from build123d import *

# Parameters (mm, degrees)
SKETCH1_W           = 66
SKETCH1_H           = 58.3
SKETCH1_R           = 2.05
BOSS_EXTRUDE1_DEPTH = 29
CUT_EXTRUDE1_START  = -29
CUT_EXTRUDE1_DEPTH  = 20
SKETCH6_W           = 10
SKETCH6_H           = 7.9
SKETCH6_R           = 2.05
BOSS_EXTRUDE2_DEPTH = 3
BOSS_EXTRUDE4_DEPTH = 7.9
BOSS_EXTRUDE5_START = -50.4
BOSS_EXTRUDE5_DEPTH = 7.9
CUT_EXTRUDE4_START  = -58.3
SKETCH8_R           = 4.05
CUT_EXTRUDE4_DEPTH  = 58.3
CUT_EXTRUDE5_REACH  = 80.031
SKETCH10_W          = 3
SKETCH10_H          = 6
SKETCH10_W_2        = 4.2
SKETCH10_W_3        = 0.4
SKETCH10_H_2        = 7.617508416
CUT_EXTRUDE6_REACH  = 84.74
SKETCH11_R          = 1.55
CUT_EXTRUDE7_DEPTH  = 2.5
BOSS_EXTRUDE6_DEPTH = 21.2
SKETCH14_R          = 2.05
BOSS_EXTRUDE7_DEPTH = 3
BOSS_EXTRUDE8_START = -4
SKETCH15_R          = 2.85
SKETCH15_R_2        = 2.05
BOSS_EXTRUDE8_DEPTH = 1
BOSS_EXTRUDE9_START = -24.2
SKETCH15_2_R        = 2.85
SKETCH15_2_R_2      = 2.05
BOSS_EXTRUDE9_DEPTH = 1


with BuildPart() as part:
    # Sketch1 → Boss-Extrude1 (new body)
    with BuildSketch(Plane(origin=(0, 0, 0), x_dir=(1, 0, 0), z_dir=(0, 1, 0))):
        Rectangle(SKETCH1_W, SKETCH1_H)
        with Locations(Location((-3.85, 0, 0), (0, 0, 90))):
            Circle(SKETCH1_R, mode=Mode.SUBTRACT)
    extrude(amount=BOSS_EXTRUDE1_DEPTH)

    # Sketch3 → Cut-Extrude1 (cut)
    with BuildSketch(Plane(origin=(0, 29, 0), x_dir=(1, 0, 0), z_dir=(0, 1, 0)).offset(CUT_EXTRUDE1_START)):
        Polygon((-33, 21.25), (-33, -21.25), (17.4, -21.25), (17.4, 21.25), (-25.1, 21.25), align=None)
    extrude(amount=CUT_EXTRUDE1_DEPTH, mode=Mode.SUBTRACT)

    # Sketch6 → Boss-Extrude2 (add)
    # profile 1 of 4: a face of its own
    with BuildSketch(Plane.XZ):
        with Locations((-38, 25.2)):
            Rectangle(SKETCH6_W, SKETCH6_H)
        with Locations(Location((-39.3, 25.2, 0), (0, 0, 270))):
            Circle(SKETCH6_R, mode=Mode.SUBTRACT)
    # profile 2 of 4: a face of its own
    with BuildSketch(Plane.XZ):
        with Locations((-38, -25.2)):
            Rectangle(SKETCH6_W, SKETCH6_H)
        with Locations(Location((-39.3, -25.2, 0), (0, 0, 270))):
            Circle(SKETCH6_R, mode=Mode.SUBTRACT)
    # profile 3 of 4: a face of its own
    with BuildSketch(Plane.XZ):
        with Locations((38, 25.2)):
            Rectangle(SKETCH6_W, SKETCH6_H)
        with Locations(Location((39.3, 25.2, 0), (0, 0, 270))):
            Circle(SKETCH6_R, mode=Mode.SUBTRACT)
    # profile 4 of 4: a face of its own
    with BuildSketch(Plane.XZ):
        with Locations((38, -25.2)):
            Rectangle(SKETCH6_W, SKETCH6_H)
        with Locations(Location((39.3, -25.2, 0), (0, 0, 270))):
            Circle(SKETCH6_R, mode=Mode.SUBTRACT)
    extrude(amount=-BOSS_EXTRUDE2_DEPTH)

    # Sketch7 → Boss-Extrude4 (add)
    with BuildSketch(Plane(origin=(0, 0, -29.15), x_dir=(-1, 0, 0), z_dir=(0, 0, -1))):
        with BuildLine():
            ThreePointArc((35.5, 3), (33.732233047, 3.732233047), (33, 5.5))
            Line((33, 5.5), (33, 3))
            Line((33, 3), (35.5, 3))
        make_face()
        with BuildLine():
            ThreePointArc((-33, 6), (-33.878679656, 3.878679656), (-36, 3))
            Line((-36, 3), (-33, 3))
            Line((-33, 3), (-33, 6))
        make_face()
    extrude(amount=-BOSS_EXTRUDE4_DEPTH)

    # Sketch7<5> → Boss-Extrude5 (add)
    with BuildSketch(Plane(origin=(0, 0, -29.15), x_dir=(-1, 0, 0), z_dir=(0, 0, -1)).offset(BOSS_EXTRUDE5_START)):
        with BuildLine():
            ThreePointArc((35.5, 3), (33.732233047, 3.732233047), (33, 5.5))
            Line((33, 5.5), (33, 3))
            Line((33, 3), (35.5, 3))
        make_face()
        with BuildLine():
            ThreePointArc((-33, 6), (-33.878679656, 3.878679656), (-36, 3))
            Line((-36, 3), (-33, 3))
            Line((-33, 3), (-33, 6))
        make_face()
    extrude(amount=-BOSS_EXTRUDE5_DEPTH)

    # Sketch8 → Cut-Extrude4 (cut)
    with BuildSketch(Plane.XY.offset(29.15).offset(CUT_EXTRUDE4_START)):
        with Locations(Location((26.05, 18, 0), (0, 0, 180))):
            Circle(SKETCH8_R)
    extrude(amount=CUT_EXTRUDE4_DEPTH, mode=Mode.SUBTRACT)

    # Sketch10 → Cut-Extrude5 (cut, up to next)
    with BuildSketch(Plane(origin=(0, 0, -29.15), x_dir=(-1, 0, 0), z_dir=(0, 0, -1)), mode=Mode.PRIVATE) as cut_extrude5_sk1:
        with Locations((-21.8, 26)):
            Rectangle(SKETCH10_W, SKETCH10_H)
    cut_extrude5_tool1 = extrude(cut_extrude5_sk1.sketch, amount=-CUT_EXTRUDE5_REACH, mode=Mode.PRIVATE) & part.part
    # Sketch10 → Cut-Extrude5 (cut, up to next)
    with BuildSketch(Plane(origin=(0, 0, -29.15), x_dir=(-1, 0, 0), z_dir=(0, 0, -1)), mode=Mode.PRIVATE) as cut_extrude5_sk2:
        with Locations((-30.9, 26)):
            Rectangle(SKETCH10_W_2, SKETCH10_H)
    cut_extrude5_tool2 = extrude(cut_extrude5_sk2.sketch, amount=-CUT_EXTRUDE5_REACH, mode=Mode.PRIVATE) & part.part
    # Sketch10 → Cut-Extrude5 (cut, up to next)
    with BuildSketch(Plane(origin=(0, 0, -29.15), x_dir=(-1, 0, 0), z_dir=(0, 0, -1)), mode=Mode.PRIVATE) as cut_extrude5_sk3:
        with Locations((-26.05, 25.191245792)):
            Rectangle(SKETCH10_W_3, SKETCH10_H_2)
    cut_extrude5_tool3 = extrude(cut_extrude5_sk3.sketch, amount=-CUT_EXTRUDE5_REACH, mode=Mode.PRIVATE) & part.part
    add(cut_extrude5_tool1.solids().sort_by_distance((21.8, 26, -29.15))[0], mode=Mode.SUBTRACT)
    add(cut_extrude5_tool2.solids().sort_by_distance((30.9, 26, -29.15))[0], mode=Mode.SUBTRACT)
    add(cut_extrude5_tool3.solids().sort_by_distance((26.05, 25.191246, -29.15))[0], mode=Mode.SUBTRACT)

    # Cut-Extrude6: up to this face of the body (flat: up to its plane)
    cut_extrude6_end = Plane(part.part.faces().sort_by_distance((23.3, 26, 0))[0])
    # Sketch11 → Cut-Extrude6 (cut, up to the picked face)
    with BuildSketch(Plane(origin=(28.8, 0, 0), x_dir=(0, 0, -1), z_dir=(1, 0, 0)), mode=Mode.PRIVATE) as cut_extrude6_sk1:
        with Locations((-21.15, 25.6)):
            Circle(SKETCH11_R)
    cut_extrude6_tool1 = split(extrude(cut_extrude6_sk1.sketch, amount=-CUT_EXTRUDE6_REACH, mode=Mode.PRIVATE), bisect_by=cut_extrude6_end, keep=Keep.BOTH, mode=Mode.PRIVATE)
    # Sketch11 → Cut-Extrude6 (cut, up to the picked face)
    with BuildSketch(Plane(origin=(28.8, 0, 0), x_dir=(0, 0, -1), z_dir=(1, 0, 0)), mode=Mode.PRIVATE) as cut_extrude6_sk2:
        with Locations((21.15, 25.6)):
            Circle(SKETCH11_R)
    cut_extrude6_tool2 = split(extrude(cut_extrude6_sk2.sketch, amount=-CUT_EXTRUDE6_REACH, mode=Mode.PRIVATE), bisect_by=cut_extrude6_end, keep=Keep.BOTH, mode=Mode.PRIVATE)
    add(cut_extrude6_tool1.solids().sort_by(Axis((28.8, 25.6, 21.15), (-1, 0, 0)))[0], mode=Mode.SUBTRACT)
    add(cut_extrude6_tool2.solids().sort_by(Axis((28.8, 25.6, -21.15), (-1, 0, 0)))[0], mode=Mode.SUBTRACT)

    # Sketch12 → Cut-Extrude7 (cut)
    with BuildSketch(Plane.XZ.offset(-20)):
        Polygon((-7.95, 0), (-5.9, -3.550704156), (-1.8, -3.550704156), (0.25, 0), (-1.8, 3.550704156), (-5.9, 3.550704156), align=None)
    extrude(amount=-CUT_EXTRUDE7_DEPTH, mode=Mode.SUBTRACT)

    # Sketch13 → Boss-Extrude6 (add)
    with BuildSketch(Plane(origin=(0, 29, 0), x_dir=(1, 0, 0), z_dir=(0, 1, 0))):
        with BuildLine():
            Line((-13.35, 9.5), (-13.35, 12.7))
            Line((-13.35, 12.7), (4.65, 12.7))
            ThreePointArc((4.65, 12.7), (7.619848481, 11.469848481), (8.85, 8.5))
            Line((8.85, 8.5), (8.85, -9.5))
            Line((8.85, -9.5), (5.65, -9.5))
            Line((5.65, -9.5), (5.65, 6.3))
            ThreePointArc((5.65, 6.3), (4.7127417, 8.5627417), (2.45, 9.5))
            Line((2.45, 9.5), (-13.35, 9.5))
        make_face()
    extrude(amount=BOSS_EXTRUDE6_DEPTH)

    # Sketch14 → Boss-Extrude7 (add)
    with BuildSketch(Plane(origin=(0, 50.2, 0), x_dir=(1, 0, 0), z_dir=(0, 1, 0))):
        with BuildLine():
            Line((-13.35, 12.7), (4.65, 12.7))
            ThreePointArc((4.65, 12.7), (7.619848481, 11.469848481), (8.85, 8.5))
            Line((8.85, 8.5), (8.85, -9.5))
            Line((8.85, -9.5), (-13.35, -9.5))
            Line((-13.35, -9.5), (-13.35, 12.7))
        make_face()
        with Locations(Location((-3.85, 0, 0), (0, 0, 90))):
            Circle(SKETCH14_R, mode=Mode.SUBTRACT)
    extrude(amount=BOSS_EXTRUDE7_DEPTH)

    # Sketch15 → Boss-Extrude8 (add)
    with BuildSketch(Plane(origin=(0, 53.2, 0), x_dir=(1, 0, 0), z_dir=(0, 1, 0)).offset(BOSS_EXTRUDE8_START)):
        with Locations(Location((-3.85, 0, 0), (0, 0, 270))):
            Circle(SKETCH15_R)
        with Locations(Location((-3.85, 0, 0), (0, 0, 90))):
            Circle(SKETCH15_R_2, mode=Mode.SUBTRACT)
    extrude(amount=BOSS_EXTRUDE8_DEPTH)

    # Sketch15<2> → Boss-Extrude9 (add)
    with BuildSketch(Plane(origin=(0, 53.2, 0), x_dir=(1, 0, 0), z_dir=(0, 1, 0)).offset(BOSS_EXTRUDE9_START)):
        with Locations(Location((-3.85, 0, 0), (0, 0, 270))):
            Circle(SKETCH15_2_R)
        with Locations(Location((-3.85, 0, 0), (0, 0, 90))):
            Circle(SKETCH15_2_R_2, mode=Mode.SUBTRACT)
    extrude(amount=BOSS_EXTRUDE9_DEPTH)


solid = part.part
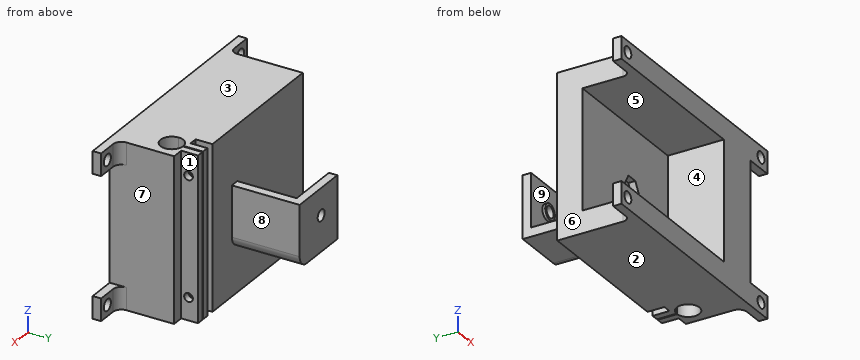
Part model, mm, in its own coordinate system. Face numbers are marked on the shaded views. A direction names the side the tool comes from. Give positions to 0.01 mm unless a question says otherwise; leave off trailing zeros. Order: outer loops, then holes, each group sorted by start corner. A loop starts at its lowest first (then second) coordinate and runs counter-clockwise, first axis right, second up. Notation, with made-up numbers: (-31, -14.75) -> (-5, -14.75) arc R9 cw to (-5, -8.75) -> close; hole circle Ø2 at (84, 33). An arc over 180 degrees is marked (long way). Use one line per item in the form item = value.
(1) Drill centre lines: line 1 (X direction, y = 24, z = -6.5); line 2 (Z direction, x = 5, y = 4.5). Where is each one in solid material? Low to high. Write a range as from..to.
Solution:
line_1 = -33..20.3, 23.3..25.85, 26.25..28.8
line_2 = -29.15..-21.25, 21.25..29.15
(2) Saw through at C-C (x = -3.85). Count the separate pieces of the cut face and the enclosed holes in it, then the cut area to 3 significant figures.
Solution:
separate_pieces = 3
enclosed_holes = 0
area = 922 mm²
(3) Saw through at D-D (y = 9.5). Write the cut outline in (x, z).
Solution:
outline = (-33, -29.15) -> (33, -29.15) -> (33, 29.15) -> (-33, 29.15) -> (-33, 21.25) -> (17.4, 21.25) -> (17.4, -21.25) -> (-33, -21.25) -> close
(4) Flat gauge pins, fed straight in: P1, Ø3, axis at y = 25.5, z = -11, coming from the +X side; P2, Ø12.5, axis at x = -4, y = 37.5, coming from the +Z side; P3, Ø4, axis at x = -17, y = 38.5, coming from the -Z side; P4, Ø7.5, axis at y = 24.5, z = -14, coming from the +X side. Where does each tip first touch, or does it go through?
Solution:
P1 = 28.8
P2 = -9.5
P3 = through
P4 = 33
(5) Pull direction Z, two halves, no side cores. Call the marked faces 1, 2, 3 and 4: +Z half, -Z half, draft (parallel to the pull), parting line (faces both ways), or undercut.
Solution:
face_1 = draft
face_2 = -Z half
face_3 = +Z half
face_4 = undercut
(6) Saw through at B-B (z = -25.2). Write the cut outline in (x, y).
Solution:
outline = (-43, 0) -> (-41.35, 0) -> (-41.35, 3) -> (-43, 3) -> close; (-37.25, 0) -> (37.25, 0) -> (37.25, 3) -> (36, 3) arc R3 cw to (33, 6) -> (33, 23) -> (28.8, 23) -> (28.8, 29) -> (26.25, 29) -> (26.25, 22.05) arc R4.05 cw (long way) to (25.85, 22.05) -> (25.85, 29) -> (23.3, 29) -> (23.3, 23) -> (20.3, 23) -> (20.3, 29) -> (-33, 29) -> (-33, 5.5) arc R2.5 cw to (-35.5, 3) -> (-37.25, 3) -> close; (41.35, 0) -> (43, 0) -> (43, 3) -> (41.35, 3) -> close
(7) Saw through at A-A (x = 39.3). Write the cut outline in (y, z).
Solution:
outline = (0, -29.15) -> (3, -29.15) -> (3, -27.25) -> (0, -27.25) -> close; (0, -23.15) -> (3, -23.15) -> (3, -21.25) -> (0, -21.25) -> close; (0, 21.25) -> (3, 21.25) -> (3, 23.15) -> (0, 23.15) -> close; (0, 27.25) -> (3, 27.25) -> (3, 29.15) -> (0, 29.15) -> close
(8) Tool access for the marked faces 5, 6, 7, 8 and 9: list every direction of +Z, -Z, +X, -X, +Y, -Y with a clear straight run to the whole face (end or side of a thin tool).
Solution:
face_5 = -X, -Y
face_6 = +Z, -Z, -X, +Y
face_7 = +X, +Y
face_8 = +Z, -Z, +X, +Y
face_9 = none
